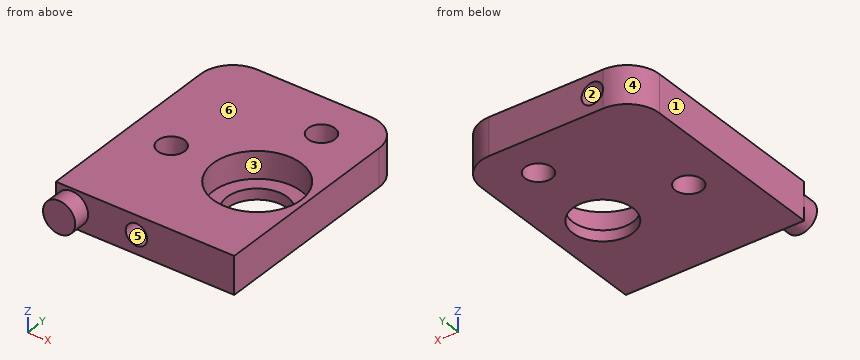
```python
from build123d import *

# Parameters (mm, degrees)
SKETCH_1_W          = 16.6
SKETCH_1_H          = 21
SKETCH_1_R          = 4.1
SKETCH_1_R_2        = 1.25
EXTRUDE_1_DEPTH     = 3.5
SKETCH_1_3_R        = 4.1
SKETCH_1_3_R_2      = 2.8
EXTRUDE_2_DEPTH     = 1
FILLET_1_R          = 3
FILLET_2_R          = 3
SKETCH_2_R          = 1
CUT_EXTRUDE_1_DEPTH = 6
SKETCH_2_3_R        = 1.5
EXTRUDE_3_DEPTH     = 1.6
SKETCH_3_R          = 1
CUT_EXTRUDE_2_DEPTH = 6


with BuildPart() as part:
    # Sketch 1 → Extrude 1 (new body)
    with BuildSketch(Plane.XY):
        with Locations((-3.7, 1.5)):
            Rectangle(SKETCH_1_W, SKETCH_1_H)
        Circle(SKETCH_1_R, mode=Mode.SUBTRACT)
        with Locations((0, 8)):
            Circle(SKETCH_1_R_2, mode=Mode.SUBTRACT)
        with Locations((-8, 0)):
            Circle(SKETCH_1_R_2, mode=Mode.SUBTRACT)
    extrude(amount=EXTRUDE_1_DEPTH)

    # Sketch 1_3 → Extrude 2 (add)
    with BuildSketch(Plane.XY):
        Circle(SKETCH_1_3_R)
        Circle(SKETCH_1_3_R_2, mode=Mode.SUBTRACT)
    extrude(amount=EXTRUDE_2_DEPTH)

    # Fillet 1
    fillet_1_edges = [part.edges().sort_by_distance(p)[0] for p in [
        (-12, 12, 1.75),
    ]]
    fillet(fillet_1_edges, radius=FILLET_1_R)

    # Fillet 2
    fillet_2_edges = [part.edges().sort_by_distance(p)[0] for p in [
        (4.6, 12, 1.75),
    ]]
    fillet(fillet_2_edges, radius=FILLET_2_R)

    # Sketch 2 → Cut-Extrude 1 (cut)
    with BuildSketch(Plane.XZ.offset(9)):
        with Locations(Location((-4.5, 1.75, 0), (0, 0, 270))):
            Circle(SKETCH_2_R)
    extrude(amount=-CUT_EXTRUDE_1_DEPTH, mode=Mode.SUBTRACT)

    # Sketch 2_3 → Extrude 3 (add)
    with BuildSketch(Plane.XZ.offset(9)):
        with Locations(Location((-10.5, 1.75, 0), (0, 0, 180))):
            Circle(SKETCH_2_3_R)
    extrude(amount=EXTRUDE_3_DEPTH)

    # Sketch 3 → Cut-Extrude 2 (cut)
    with BuildSketch(Plane(origin=(0, 12, 0), x_dir=(1, 0, 0), z_dir=(0, 1, 0))):
        with Locations(Location((-8, -1.75, 0), (0, 0, 270))):
            Circle(SKETCH_3_R)
    extrude(amount=-CUT_EXTRUDE_2_DEPTH, mode=Mode.SUBTRACT)


solid = part.part
```
Geometry check sheet. Reference: the model listing, model coordinates, mm. Face numbers are marked on the shaded views. A direction names the side the tool comes from. Coordinates: 2 decimals unless noted, no trailing zeros. Loops run counter-clockwise (first coordinate to the right, second up) from the corner with the lowest first, then second, coordinate; pieces in that order, holes last. Notation, with made-up numbers: (10, 39) - (34, 39) arc R21 cw to (34, 56) - close; hole circle Ø11 at (22, 54). An arc over 180 degrees is marked (long way). One line per item, written item: value. Start each with the question number.
(1) Cross-section at B-B on x = -8. Enter the section's corners in (y, z).
(2) Cross-section at D-D on y = 0. Enter the section's corners in (x, z).
(3) Tool access check on the marked faces 1, 2 and 3. Record the directions out of +Z, -Z, +X, -X, +Y, -Y that give a thin tool (end or side, any length) a straight path to the whole face; none if there is none.
(4) Cross-section at C-C on x = 0. Enter the section's corners in (y, z).
(5) Material ranges on line 1 (Y direction, x = 0, z = 0.45); line 2 (Y direction, x = 0, z = 2.65); line 3 (X direction, y = 8.75, z = 2.6), recorded low to high. Write a range as [from, to].
(6) Mould release check, pull along Z, two halves, no side actions. Record for the marked faces 4, 5 and 6: released by +Z, released by -Z, zero draft, split by the parting line, or undercut.
(7) Depth check by flat-ended pin: P1, Ø6.5, axis at x = 0, y = 0, coming from the -Z side; P2, Ø0.6, axis at x = -8.5, z = 1.5, coming from the +Y side; P3, Ø1.5, axis at x = 0, y = 8, coming from the -Z side; P4, Ø0.6, axis at x = -4, z = 2, coming from the -Y side. Enter the tip coordinate at first touch or a pass-through.
(8) Cross-section at A-A on y = 8. Enter the section's corners in (x, z), plus the area to 3 significant figures.
Results below:
1. outline: (-9, 0) - (-1.25, 0) - (-1.25, 3.5) - (-9, 3.5) - close; (1.25, 0) - (12, 0) - (12, 0.75) - (6, 0.75) - (6, 2.75) - (12, 2.75) - (12, 3.5) - (1.25, 3.5) - close
2. outline: (-12, 0) - (-9.25, 0) - (-9.25, 3.5) - (-12, 3.5) - close; (-6.75, 0) - (-2.8, 0) - (-2.8, 1) - (-4.1, 1) - (-4.1, 3.5) - (-6.75, 3.5) - close; (2.8, 0) - (4.6, 0) - (4.6, 3.5) - (4.1, 3.5) - (4.1, 1) - (2.8, 1) - close
3. face 1: +Z, -Z, -X, +Y, -Y
3. face 2: +Y
3. face 3: +Z
4. outline: (-9, 0) - (-2.8, 0) - (-2.8, 1) - (-4.1, 1) - (-4.1, 3.5) - (-9, 3.5) - close; (2.8, 0) - (6.75, 0) - (6.75, 3.5) - (4.1, 3.5) - (4.1, 1) - (2.8, 1) - close; (9.25, 0) - (12, 0) - (12, 3.5) - (9.25, 3.5) - close
5. line 1: y = [-9, -2.8], [2.8, 6.75], [9.25, 12]
5. line 2: y = [-9, -4.1], [4.1, 6.75], [9.25, 12]
5. line 3: x = [-12, -8.53], [-7.47, -1], [1, 4.6]
6. face 4: zero draft
6. face 5: undercut
6. face 6: released by +Z
7. P1: stops at z = 0
7. P2: stops at y = 6
7. P3: passes through
7. P4: stops at y = -3
8. outline: (-12, 0) - (-1.25, 0) - (-1.25, 3.5) - (-12, 3.5) - close; (1.25, 0) - (4.6, 0) - (4.6, 3.5) - (1.25, 3.5) - close; hole circle Ø2 at (-8, 1.75)
8. area: 46.2 mm2
